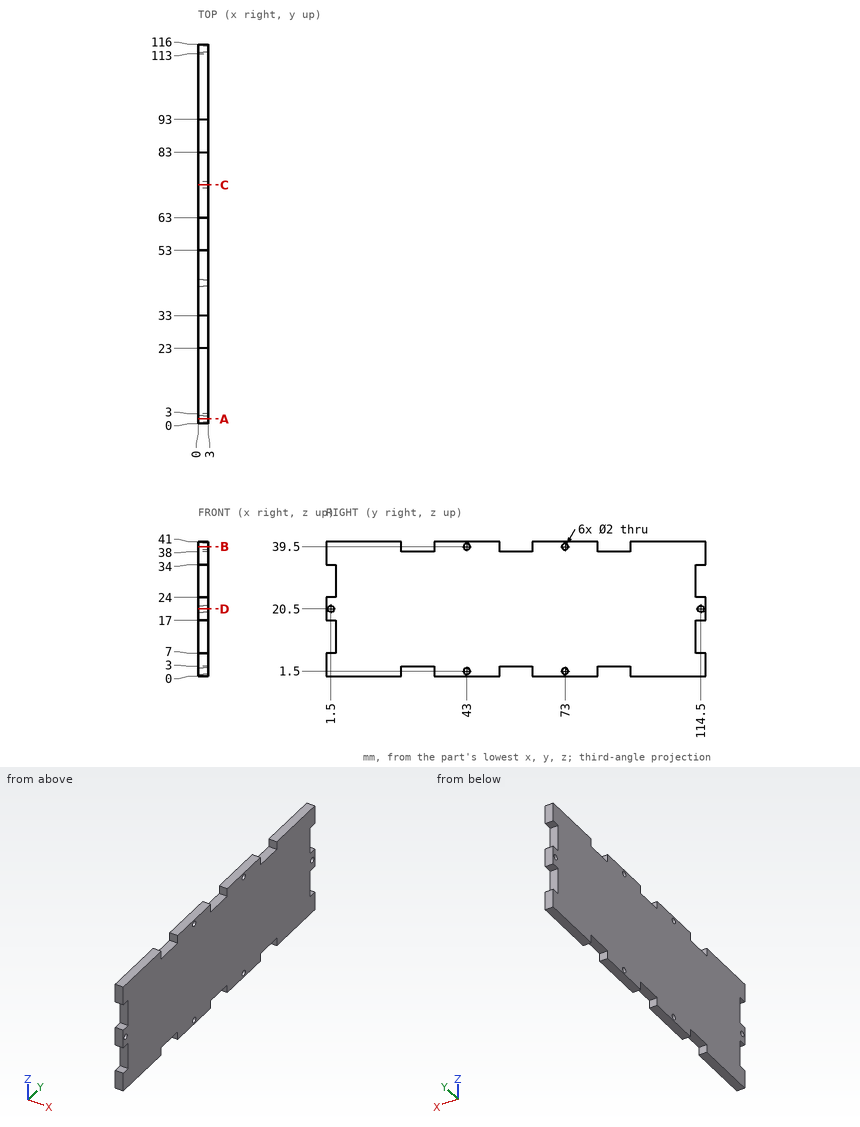
Part print with two shaded views. Sizes in mm from the minimum x, y, z corner. Coordinates: 2 decimals unless noted, no trailing zeros. Write each loop counter-clockwise with the first axis right and the second up, starting at its lowest first coordinate (ties: lowest second). Pieces come first, ordered by that corner, then holes.
(1) Cut at A-A on y = 1.5. List the corners of the cut face in (x, z).
(2) Cut at C-C on y = 73. List the corners of the cut face in (x, z).
(3) Drill centre lines: line 1 (Z direction, x = 0.95, y = 43); line 2 (Z direction, x = 1.15, y = 114.5); line 3 (Y direction, x = 0.8, z = 20.5). Where is each one in solid material? Low to high.
(4) Pin check, flat tip, straight feed: pin 1 Ø0.9 at (x, y) = (1, 29.5) entering from -Z. Stop position of the tip, or through.
(5) Cut at B-B on z = 39.5. List the corners of the cut face in (x, y), and give its area (3 significant figures).
(6) Cut at D-D on z = 20.5. List the corners of the cut face in (x, y), and give its area (3 significant figures).
Working result:
1. outline: (0, 0) - (3, 0) - (3, 7) - (0, 7) - close; (0, 17) - (3, 17) - (3, 19.5) - (0, 19.5) - close; (0, 21.5) - (3, 21.5) - (3, 24) - (0, 24) - close; (0, 34) - (3, 34) - (3, 41) - (0, 41) - close
2. outline: (0, 0) - (3, 0) - (3, 0.5) - (0, 0.5) - close; (0, 2.5) - (3, 2.5) - (3, 38.5) - (0, 38.5) - close; (0, 40.5) - (3, 40.5) - (3, 41) - (0, 41) - close
3. line 1: z = 0 to 0.5, 2.5 to 38.5, 40.5 to 41
3. line 2: z = 0 to 7, 17 to 19.5, 21.5 to 24, 34 to 41
3. line 3: y = 0 to 0.5, 2.5 to 113.5, 115.5 to 116
4. pin 1: stops at z = 3
5. outline: (0, 0) - (3, 0) - (3, 23) - (0, 23) - close; (0, 33) - (3, 33) - (3, 42) - (0, 42) - close; (0, 44) - (3, 44) - (3, 53) - (0, 53) - close; (0, 63) - (3, 63) - (3, 72) - (0, 72) - close; (0, 74) - (3, 74) - (3, 83) - (0, 83) - close; (0, 93) - (3, 93) - (3, 116) - (0, 116) - close
5. area: 246 mm2
6. outline: (0, 0) - (3, 0) - (3, 0.5) - (0, 0.5) - close; (0, 2.5) - (3, 2.5) - (3, 113.5) - (0, 113.5) - close; (0, 115.5) - (3, 115.5) - (3, 116) - (0, 116) - close
6. area: 336 mm2
